```python
from build123d import *

# Parameters (mm, degrees)
EXTRUSION1_DEPTH           = 60
ESQUISSE2_R                = 1.5
EXTRUSION2_DEPTH           = 60
ESQUISSE3_R                = 1.5
EXTRUSION3_DEPTH           = 60
R_P_TITION_LIN_AIRE1_COUNT = 2
R_P_TITION_LIN_AIRE1_PITCH = 40


with BuildPart() as part:
    # Esquisse1 → Extrusion1 (new body)
    with BuildSketch(Plane.XY):
        Polygon((0, 0), (1.5, 0), (15, 0), (15, 1.5), (1.5, 1.5), (1.5, 15), (0, 15), align=None)
    extrude(amount=EXTRUSION1_DEPTH)

    # Esquisse2 → Extrusion2 (cut)
    with BuildSketch(Plane.ZY):
        with Locations((30, 10)):
            Circle(ESQUISSE2_R)
    extrude(amount=-EXTRUSION2_DEPTH, mode=Mode.SUBTRACT)

    # Esquisse3 → Extrusion3 (cut)
    with BuildSketch(Plane.XZ):
        with Locations(Location((10, 10, 0), (0, 0, 270))):
            Circle(ESQUISSE3_R)
    extrusion3 = extrude(amount=-EXTRUSION3_DEPTH, mode=Mode.SUBTRACT)

    # Répétition linéaire1: Extrusion3 ×2
    with Locations(*[(0, 0, i * R_P_TITION_LIN_AIRE1_PITCH) for i in range(1, R_P_TITION_LIN_AIRE1_COUNT)]):
        add(extrusion3, mode=Mode.SUBTRACT)


solid = part.part
```
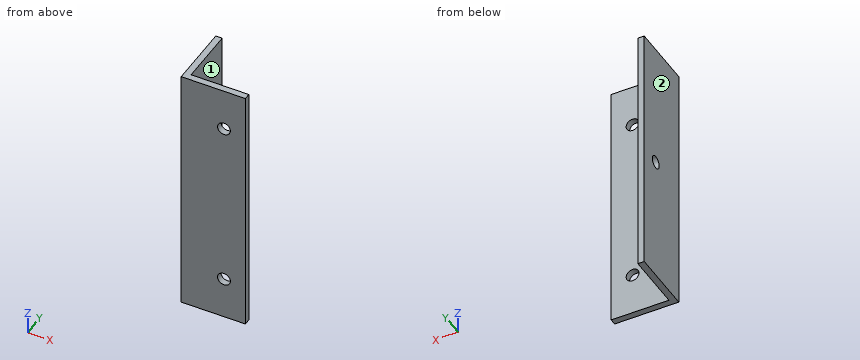
The listing builds one solid part. Answer for the finished solid, in the listing's coordinates (mm). Face numbers are marked on the shaded views. A direction names the side the tool comes from. Give positions to 0.01 mm unless a question says otherwise; leave off trailing zeros. Order: outer loops, then holes, each group sorted by start corner. A loop starts at its lowest first (then second) coordinate and runs counter-clockwise, first axis right, second up. Notation, with made-up numbers: M -10.75,-36.75 L 16.25,-36.75 A23 cw 16.25,-10.75 Z; hole C 16,-8.5 d5. An arc over 180 degrees is marked long. Put each result on its own line as item: value. Start each with the question number.
Item 1: The part is cut by section C-C, the plane y = 10. Determine the outline of the cut face in (x, z), and give its area (3 significant figures).
Item 2: Find the intervals of material crossed by line 1 along Y through (x, z) = (0.9, 30); line 2 along Y through (x, z) = (8.75, 37.5), in increasing order.
Item 3: The part is cut by section D-D, the plane z = 37. Determine the outline of the cut face in (x, y).
Item 4: Which of the six approach directions +Z, -Z, +X, -X, +Y, -Y give full straight-line access (tool end or side, diameter ignored) to the marked faces 1 and 2?
Item 5: The part is cut by section A-A, the plane x = 10. Determine the outline of the cut face in (y, z), and give its area (3 significant figures).
Item 6: The part is cut by section B-B, the plane z = 50. Determine the outline of the cut face in (x, y), and give its area (4 significant figures).
Item 7: A flat-ended cylindrical pin translates along its axis: P1, Ø4, axis at x = 4.5, z = 37, coming from the +Y side. Find the tip coordinate at first contact, or state that the pin passes through.
Answer key:
1. outline: M 0,0 L 1.5,0 L 1.5,28.5 L 0,28.5 Z; M 0,31.5 L 1.5,31.5 L 1.5,60 L 0,60 Z
1. area: 85.5 mm²
2. line 1: y = 0 to 8.5, 11.5 to 15
2. line 2: y = 0 to 1.5
3. outline: M 0,0 L 15,0 L 15,1.5 L 1.5,1.5 L 1.5,15 L 0,15 Z
4. face 1: +Z, -Z, +X, +Y
4. face 2: +Z, -Z, -X, +Y, -Y
5. outline: M 0,0 L 1.5,0 L 1.5,8.5 L 0,8.5 Z; M 0,11.5 L 1.5,11.5 L 1.5,48.5 L 0,48.5 Z; M 0,51.5 L 1.5,51.5 L 1.5,60 L 0,60 Z
5. area: 81.0 mm²
6. outline: M 0,0 L 8.5,0 L 8.5,1.5 L 1.5,1.5 L 1.5,15 L 0,15 Z; M 11.5,0 L 15,0 L 15,1.5 L 11.5,1.5 Z
6. area: 38.25 mm²
7. P1: stops at y = 1.5
